Check sheet for the drawn part. Datum: minimum x, y, z corner. Units: mm. A direction names the side the tool comes from. Give positions to 0.01 mm unless a question says otherwise; leave off trailing zeros. Order: outer loops, then holes, each group sorted by start corner. A loop starts at its lowest first (then second) coordinate and runs counter-clockwise, first axis right, second up. Notation, with made-up numbers: (72.25, 59.5) -> (78.25, 59.5) arc R13 cw to (78.25, 72.5) -> close; hole circle Ø5 at (13.5, 50). An arc over 180 degrees is marked (long way). Answer in a Markdown table with one row per item. Add a question column.
(1) Thickness scan on L1, parallel to Y at x = 35, z = 50; L2, parallel to Z at x = 20, y = 50; L3, parallel to X at y = 49, z = 39.5. Record the ranges inside material, lowest first. Write a range as [from, to].
(2) Go/stop test with flat-tipped pins: pin 1 (1.5 mm diameter, centred on x = 74.5, z = 38, fed in from -Y); pin 2 (1.5 mm diameter, centred on x = 59, z = 52, fed in from +Y); pin 3 (4 mm diameter, centred on x = 15, z = 30, fed in from -Y). Record where each tip stops, or that it passes through.
(3) Set-up check for the marked faces 1 and 2: record each of +Z, -Z, +X, -X, +Y, -Y from which the full face is reachable in a straight line by a thin tool's end or side.
(4) Cross-section at A-A (y = 50.8). Record the cut outline in (x, z) (3 decimals).
(5) Cross-section at B-B (z = 50.8). Record the cut outline in (x, y) (3 decimals), then the cut area to 3 significant figures.
(6) Cross-section at C-C (x = 21.5). Record the cut outline in (y, z) (3 decimals), then the cut area to 3 significant figures.
(7) Cross-section at D-D (y = 62). Record the cut outline in (x, z).
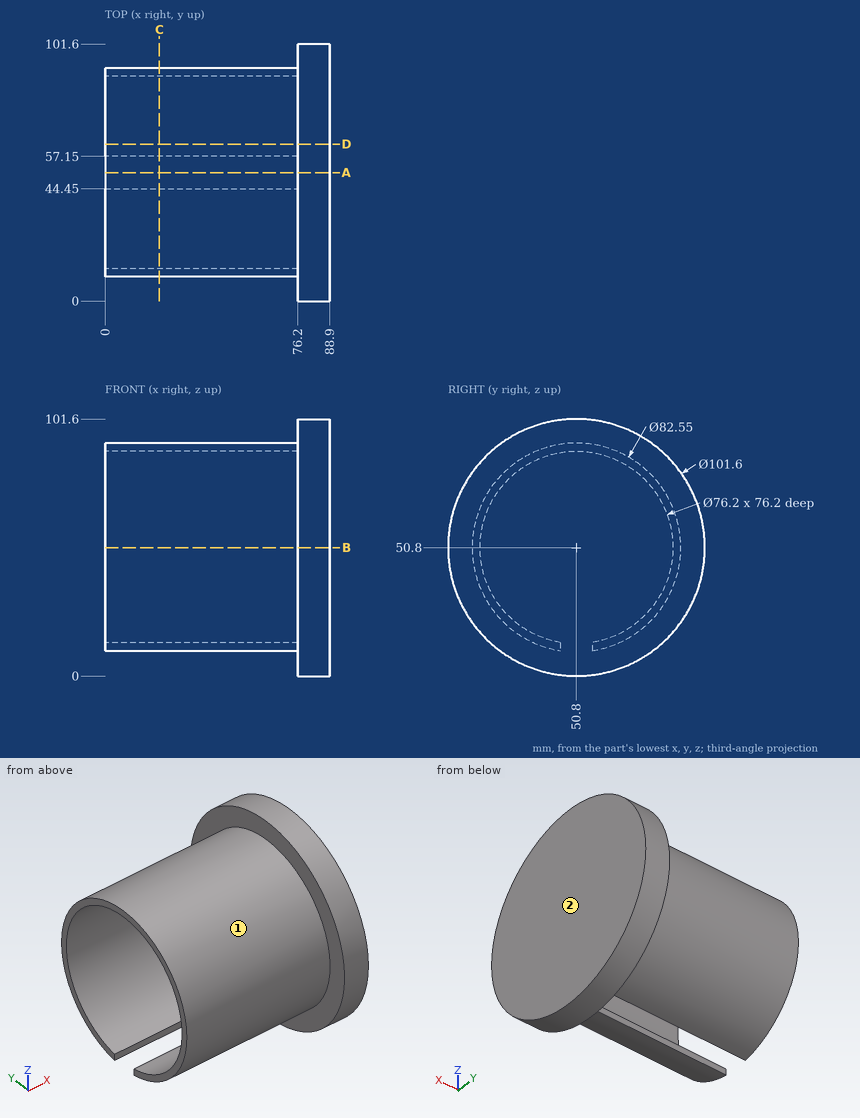
Answer below:
| question | item | result |
|---|---|---|
| 1 | L1 | y = [9.53, 12.71], [88.89, 92.07] |
| 1 | L2 | z = [88.89, 92.07] |
| 1 | L3 | x = [76.2, 88.9] |
| 2 | pin 1 | stops at y = 11.32 |
| 2 | pin 2 | stops at y = 92.07 |
| 2 | pin 3 | stops at y = 14.06 |
| 3 | face 1 | -X |
| 3 | face 2 | +Z, -Z, +X, +Y, -Y |
| 4 | outline | (0, 88.9) -> (76.2, 88.9) -> (76.2, 0) -> (88.9, 0) -> (88.9, 101.6) -> (76.2, 101.6) -> (76.2, 92.075) -> (0, 92.075) -> close |
| 5 | outline | (0, 9.525) -> (76.2, 9.525) -> (76.2, 0) -> (88.9, 0) -> (88.9, 101.6) -> (76.2, 101.6) -> (76.2, 92.075) -> (0, 92.075) -> (0, 88.9) -> (76.2, 88.9) -> (76.2, 12.7) -> (0, 12.7) -> close |
| 5 | area | 1,770 mm² |
| 6 | outline | (44.45, 10.016) -> (44.45, 13.233) arc R38.1 cw (long way) to (57.15, 13.233) -> (57.15, 10.016) arc R41.275 ccw (long way) to start |
| 6 | area | 751 mm² |
| 7 | outline | (0, 11.07) -> (76.2, 11.07) -> (76.2, 1.25) -> (88.9, 1.25) -> (88.9, 100.35) -> (76.2, 100.35) -> (76.2, 90.53) -> (0, 90.53) -> (0, 87.22) -> (76.2, 87.22) -> (76.2, 14.38) -> (0, 14.38) -> close |
